Here's how the part is built. I have some questions about the finished solid (model axes, mm). Face numbers are marked on the shaded views. Coordinates: 2 decimals unless noted, no trailing zeros. Order: outer loops, then holes, each group sorted by start corner. A loop starts at its lowest first (then second) coordinate and runs counter-clockwise, first axis right, second up. Notation, with made-up numbers: (-8.5, 53) - (10.5, 53) arc R16 cw to (10.5, 77) - close; hole circle Ø11 at (79.5, -25). An arc over 180 degrees is marked (long way). Answer in a Markdown table with one row per item. Add a question column.
Item 1: If I drill on line 1 along Y through (x, z) = (0, 0.3); line 2 along Z through (x, y) = (10.5, -15); line 3 along X through (y, z) = (-1.5, 8.5), over which ranges is the centre line in solid material (lowest first)? Write a range as from..to.
Item 2: I want a section at C-C (z = -4.5). Please give me the cut outline in (x, y).
Item 3: Thinking about a two-plate mould opening in Y: for the marked faces 1 and 2, which applies, +Y half, -Y half, draft (parallel to the pull), parting line (faces both ways), or undercut?
Item 4: I want a section at D-D (x = -4.5). Please give me the cut outline in (y, z).
Item 5: I want a section at B-B (y = 0). Please give me the cut outline in (x, z).
Item 6: Will these pins go through, and if not, where does the flat tip stop? pin 1 Ø1.5 at (x, z) = (4, 6.5) entering from +Y; pin 2 Ø6 at (x, z) = (0.5, -2.5) entering from -Y; pin 3 Ø8 at (x, z) = (-13, -3) entering from +Y.
Item 7: I want a section at A-A (x = 0). Please give me the cut outline in (y, z), plus the area to 3 significant figures.
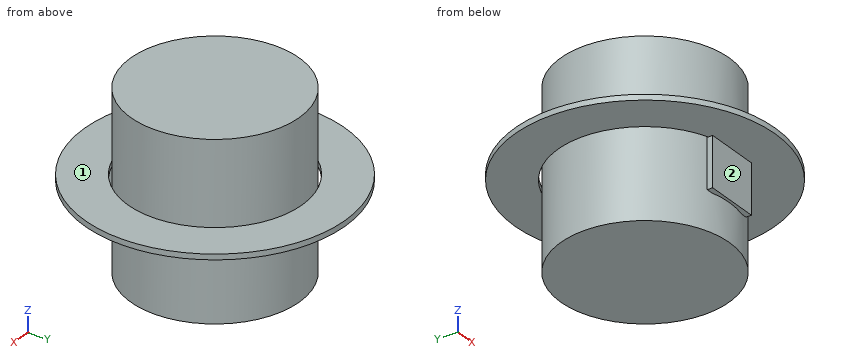
```python
from build123d import *

# Parameters (mm, degrees)
F0_R     = 19
F0_R_2   = 12.7
F1_DEPTH = 0.8
F2_W     = 8
F2_H     = 0.8
F3_DEPTH = 8
F4_R     = 12.3
F5_DEPTH = 12.7


with BuildPart() as f1:
    # F0 (on Top) → F1 (new body)
    with BuildSketch(Plane.XY):
        Circle(F0_R)
        Circle(F0_R_2, mode=Mode.SUBTRACT)
    extrude(amount=F1_DEPTH)

    # F2 (on face) → F3 (join)
    with BuildSketch(Plane.XY.offset(0.8)):
        with Locations((0, -12.3)):
            Rectangle(F2_W, F2_H)
    extrude(amount=-F3_DEPTH)

    # F4 (on Top) → F5 (join, symmetric)
    with BuildSketch(Plane.XY):
        Circle(F4_R)
    extrude(amount=F5_DEPTH, both=True)


solid = f1.part
```
Values follow:
| question | item | result |
|---|---|---|
| 1 | line 1 | y = -19..12.3, 12.7..19 |
| 1 | line 2 | z = 0..0.8 |
| 1 | line 3 | x = -12.21..12.21 |
| 2 | outline | (-4, -12.7) - (4, -12.7) - (4, -11.9) - (3.11, -11.9) arc R12.3 ccw (long way) to (-3.11, -11.9) - (-4, -11.9) - close |
| 3 | face 1 | draft |
| 3 | face 2 | -Y half |
| 4 | outline | (-18.46, 0) - (-11.88, 0) - (-11.88, 0.8) - (-18.46, 0.8) - close; (-11.45, -12.7) - (11.45, -12.7) - (11.45, 12.7) - (-11.45, 12.7) - close; (11.88, 0) - (18.46, 0) - (18.46, 0.8) - (11.88, 0.8) - close |
| 5 | outline | (-19, 0) - (-12.7, 0) - (-12.7, 0.8) - (-19, 0.8) - close; (-12.3, -12.7) - (12.3, -12.7) - (12.3, 12.7) - (-12.3, 12.7) - close; (12.7, 0) - (19, 0) - (19, 0.8) - (12.7, 0.8) - close |
| 6 | pin 1 | stops at y = 11.86 |
| 6 | pin 2 | stops at y = -19 |
| 6 | pin 3 | stops at y = 15.93 |
| 7 | outline | (-19, 0) - (-12.7, 0) - (-12.7, -7.2) - (-12.3, -7.2) - (-12.3, -12.7) - (12.3, -12.7) - (12.3, 12.7) - (-12.3, 12.7) - (-12.3, 0.8) - (-19, 0.8) - close; (12.7, 0) - (19, 0) - (19, 0.8) - (12.7, 0.8) - close |
| 7 | area | 638 mm^2 |
